Verification items for the finished model (mm, model axes). A direction names the side the tool comes from. Give positions to 0.01 mm unless a question says otherwise; leave off trailing zeros. Loops run counter-clockwise (first coordinate to the right, second up) from the corner with the lowest first, then second, coordinate; pieces in that order, holes last. Notation, with made-up numbers: (18.5, -9.75) -> (72.5, -9.75) arc R19 ccw to (72.5, 27.25) -> close; hole circle Ø9 at (2, -28.75). An arc over 180 degrees is marked (long way). Answer in a Markdown table with one row per item. Add a question column.
Q1. Section check C-C on y = 0.45. Enter the section's corners in (x, z).
Q2. Section check A-A on z = 0. Enter the section's corners in (x, y), and give its area (3 significant figures).
Q3. Set-up check for faces 1 (the face through (23, 1, 1.591)), 2 (the face through (23, 0, 0)), 3 (the face through (22, 1, -1.591)): record each of +Z, -Z, +X, -X, +Y, -Y from which the full face is reachable in a straight line by a thin tool's end or side.
Q4. Section check D-D on x = 20. Enter the section's corners in (y, z).
Q5. Material ranges on probe 1 along X at (y, z) = (1.3, -0.1); probe 2 along Z at (x, y) = (45.5, 1.65); probe 3 along X at (y, z) = (1.8, -0.4), recorded low to high.
Q6. Section check B-B on x = 0. Enter the section's corners in (y, z), and give its area (3 significant figures).
Q7. Gauge pin test, flat ends, axial feed: P1, Ø1, axis at y = 2, z = -2, coming from the +X side; P2, Ø1, axis at x = 18.5, y = 1, coming from the -Z side; P3, Ø1, axis at y = 0.5, z = -2, coming from the -X side; P4, Ø1.2, axis at x = 0, z = 0, coming from the -Y side. Record the tip position at first contact, or that the pin passes through.
```python
from build123d import *

# Parameters (mm, degrees)
SKETCH1_R           = 1
BOSS_EXTRUDE2_DEPTH = 2
FILLET2_R           = 10


with BuildPart() as part:
    # Sketch1 → Boss-Extrude2 (new body)
    with BuildSketch(Plane(origin=(0, 0, 0), x_dir=(1, 0, 0), z_dir=(0, 1, 0))):
        with BuildLine():
            Line((0.833333333, 2.357022604), (3.0003558, 1.590864463))
            Line((3.0003558, 1.590864463), (42.4996442, 1.590864463))
            Line((42.4996442, 1.590864463), (44.666666667, 2.357022604))
            ThreePointArc((44.666666667, 2.357022604), (48, 0), (44.666666667, -2.357022604))
            Line((44.666666667, -2.357022604), (42.4996442, -1.590864463))
            Line((42.4996442, -1.590864463), (3.0003558, -1.590864463))
            Line((3.0003558, -1.590864463), (0.833333333, -2.357022604))
            ThreePointArc((0.833333333, -2.357022604), (-2.5, 0), (0.833333333, 2.357022604))
        make_face()
        Circle(SKETCH1_R, mode=Mode.SUBTRACT)
        with Locations((45.5, 0)):
            Circle(SKETCH1_R, mode=Mode.SUBTRACT)
    extrude(amount=BOSS_EXTRUDE2_DEPTH)

    # Fillet2
    fillet2_edges = [part.edges().sort_by_distance(p)[0] for p in [
        (42.4996442, 1, -1.590864463),
        (42.4996442, 1, 1.590864463),
        (3.0003558, 1, 1.590864463),
        (3.0003558, 1, -1.590864463),
    ]]
    fillet(fillet2_edges, radius=FILLET2_R)


solid = part.part
```
Taken from the geometry:
| question | item | result |
|---|---|---|
| 1 | outline | (0.83, -2.36) -> (1.38, -2.16) arc R10 cw to (4.72, -1.59) -> (40.78, -1.59) arc R10 cw to (44.12, -2.16) -> (44.67, -2.36) arc R2.5 ccw (long way) to (44.67, 2.36) -> (44.12, 2.16) arc R10 cw to (40.78, 1.59) -> (4.72, 1.59) arc R10 cw to (1.38, 2.16) -> (0.83, 2.36) arc R2.5 ccw (long way) to start; hole circle Ø2 at (0, 0); hole circle Ø2 at (45.5, 0) |
| 2 | outline | (-2.5, 0) -> (-1, 0) -> (-1, 2) -> (-2.5, 2) -> close; (1, 0) -> (44.5, 0) -> (44.5, 2) -> (1, 2) -> close; (46.5, 0) -> (48, 0) -> (48, 2) -> (46.5, 2) -> close |
| 2 | area | 93.0 mm² |
| 3 | face 1 | +Z, +Y, -Y |
| 3 | face 2 | +Z, -Z, +X, -X, -Y |
| 3 | face 3 | -Z, +Y, -Y |
| 4 | outline | (0, -1.59) -> (2, -1.59) -> (2, 1.59) -> (0, 1.59) -> close |
| 5 | probe 1 | x = -2.5 to -0.99, 0.99 to 44.51, 46.49 to 48 |
| 5 | probe 2 | z = -2.5 to -1, 1 to 2.5 |
| 5 | probe 3 | x = -2.47 to -0.92, 0.92 to 44.58, 46.42 to 47.97 |
| 6 | outline | (0, -2.5) -> (2, -2.5) -> (2, -1) -> (0, -1) -> close; (0, 1) -> (2, 1) -> (2, 2.5) -> (0, 2.5) -> close |
| 6 | area | 6.00 mm² |
| 7 | P1 | stops at x = 47.5 |
| 7 | P2 | stops at z = -1.59 |
| 7 | P3 | stops at x = -2 |
| 7 | P4 | passes through |
